Work out the finished part from the listing and answer in its coordinate system (mm). Face numbers are marked on the shaded views. A direction names the side the tool comes from. Round coordinates to 2 decimals unless told otherwise and drop trailing zeros. Loops run counter-clockwise (first coordinate to the right, second up) from the corner with the lowest first, then second, coordinate; pieces in that order, holes last. Notation, with made-up numbers: (9, -2) - (26, -2) arc R6 ccw to (26, 3) - close; hole circle Ø3 at (2.25, 20). An arc over 180 degrees is marked (long way). Answer as CSV lines item,"result". Start each with the question number.
```python
from build123d import *

# Parameters (mm, degrees)
F0_W     = 33
F0_H     = 33
F1_DEPTH = 55
F2_W     = 25.027660653
F2_H     = 24.4021397084
F3_DEPTH = 14
F4_R     = 8
F5_DEPTH = 7
F7_D     = 2.5
F8_D     = 5


with BuildPart() as f1:
    # F0 (on Top) → F1 (new body)
    with BuildSketch(Plane.XY):
        Rectangle(F0_W, F0_H)
    extrude(amount=F1_DEPTH)

    # F2 (on face) → F3 (join)
    with BuildSketch(Plane.XY.offset(55)):
        Rectangle(F2_W, F2_H)
    extrude(amount=F3_DEPTH)

    # F4 (on face) → F5 (join)
    with BuildSketch(Plane(origin=(0, 0, 0), x_dir=(1, 0, 0), z_dir=(0, 0, -1))):
        Circle(F4_R)
    extrude(amount=F5_DEPTH)

    # F7 (through all)
    with Locations(Plane.XZ.offset(16.5)):
        with Locations((-8, 47.4), (0, 47.4), (8, 47.4), (8, 7.6), (0, 7.6), (-8, 7.6)):
            Hole(F7_D / 2)

    # F8 (through all)
    with Locations(Plane.XZ.offset(16.5)):
        with Locations((0, 27.5)):
            Hole(F8_D / 2)


solid = f1.part
```
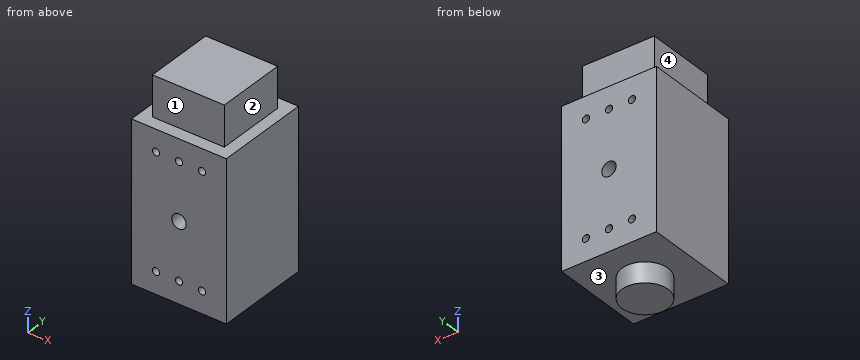
Item 1: Section C-C, the plane z = 47.4 is taken. Give the vertices of the cut face in (x, y).
Item 2: Section B-B, the plane y = 0 is taken. Give the vertices of the cut face in (x, z).
Item 3: Section D-D, the plane x = 0 is taken. Give the vertices of the cut face in (y, z).
Item 4: Flat-ended cylindrical pins translate along their axes: pin 1 Ø1.5 at (x, z) = (8, 47.4) entering from +Y; pin 2 Ø7 at (x, z) = (2.5, 61) entering from -Y; pin 3 Ø12 at (x, y) = (7, 13) entering from -Z; pin 4 Ø4 at (y, z) = (0, 64) entering from +X. Find the tip coordinate at first contact, or state that the pin passes through.
Item 5: Find the intervals of material crossed by L1, parallel to X at y = -10.5, z = 7.5; L2, parallel to Z at x = 0, y = -4; L3, parallel to Z at x = -11.5, y = 15, in increasing order.
Item 6: Which of the six approach directions +Z, -Z, +X, -X, +Y, -Y give full straight-line access (tool end or side, diameter ignored) to the marked faces 1, 2, 3 and 4?
Item 7: Section A-A, the plane z = 29 is taken. Give the vertices of the cut face in (x, y), and give its area (3 significant figures).
Answer:
1,outline,"(-16.5, -16.5) - (-9.25, -16.5) - (-9.25, 16.5) - (-16.5, 16.5) - close; (-6.75, -16.5) - (-1.25, -16.5) - (-1.25, 16.5) - (-6.75, 16.5) - close; (1.25, -16.5) - (6.75, -16.5) - (6.75, 16.5) - (1.25, 16.5) - close; (9.25, -16.5) - (16.5, -16.5) - (16.5, 16.5) - (9.25, 16.5) - close"
2,outline,"(-16.5, 0) - (-8, 0) - (-8, -7) - (8, -7) - (8, 0) - (16.5, 0) - (16.5, 55) - (12.51, 55) - (12.51, 69) - (-12.51, 69) - (-12.51, 55) - (-16.5, 55) - close; hole circle Ø2.5 at (-8, 7.6); hole circle Ø2.5 at (-8, 47.4); hole circle Ø5 at (0, 27.5); hole circle Ø2.5 at (0, 7.6); hole circle Ø2.5 at (0, 47.4); hole circle Ø2.5 at (8, 7.6); hole circle Ø2.5 at (8, 47.4)"
3,outline,"(-16.5, 0) - (-8, 0) - (-8, -7) - (8, -7) - (8, 0) - (16.5, 0) - (16.5, 6.35) - (-16.5, 6.35) - close; (-16.5, 8.85) - (16.5, 8.85) - (16.5, 25) - (-16.5, 25) - close; (-16.5, 30) - (16.5, 30) - (16.5, 46.15) - (-16.5, 46.15) - close; (-16.5, 48.65) - (16.5, 48.65) - (16.5, 55) - (12.2, 55) - (12.2, 69) - (-12.2, 69) - (-12.2, 55) - (-16.5, 55) - close"
4,pin 1,"passes through"
4,pin 2,"stops at y = -12.2"
4,pin 3,"stops at z = 0"
4,pin 4,"stops at x = 12.51"
5,L1,"x = -16.5 to -9.25, -6.75 to -1.25, 1.25 to 6.75, 9.25 to 16.5"
5,L2,"z = -7 to 6.35, 8.85 to 25, 30 to 46.15, 48.65 to 69"
5,L3,"z = 0 to 55"
6,face 1,"+Z, +X, -X, -Y"
6,face 2,"+Z, +X, +Y, -Y"
6,face 3,"-Z"
6,face 4,"+Z, -X, +Y, -Y"
7,outline,"(-16.5, -16.5) - (-2, -16.5) - (-2, 16.5) - (-16.5, 16.5) - close; (2, -16.5) - (16.5, -16.5) - (16.5, 16.5) - (2, 16.5) - close"
7,area,"957 mm²"
